CAD build for the part. Positions are in the model's coordinates, mm. Face numbers are marked on the shaded views. A direction names the side the tool comes from. Give positions to 0.01 mm unless a question says otherwise; leave off trailing zeros. Loops run counter-clockwise (first coordinate to the right, second up) from the corner with the lowest first, then second, coordinate; pieces in that order, holes last.
```python
from build123d import *

# Parameters (mm, degrees)
SKETCH1_R               = 15.875
BOSS_EXTRUDE1_DEPTH     = 9.2
SKETCH2_W               = 2.259426776
SKETCH2_H               = 16.292984729
SKETCH2_W_2             = 2.453909841
SKETCH2_H_2             = 18.61191006
CUT_EXTRUDE2_DEPTH      = 2
SKETCH3_R               = 4
BOSS_EXTRUDE3_DEPTH     = 1
BOSS_EXTRUDE4_START     = -5
BOSS_EXTRUDE4_OUTLINE_R = 1.7
BOSS_EXTRUDE4_DEPTH     = 5


# Read off the part's stored shape, not the designer's step: Boss-Extrude4
with BuildPart() as part:
    # Sketch1 → Boss-Extrude1 (new body)
    with BuildSketch(Plane(origin=(0, 0, 0), x_dir=(1, 0, 0), z_dir=(0, 1, 0))):
        with Locations(Location((0, 0, 0), (0, 0, 270))):
            Circle(SKETCH1_R)
    extrude(amount=BOSS_EXTRUDE1_DEPTH)

    # Sketch2 → Cut-Extrude2 (cut)
    with BuildSketch(Plane(origin=(0, 9.2, 0), x_dir=(1, 0, 0), z_dir=(0, 1, 0))):
        with Locations((-15.629713388, -0.847675915)):
            Rectangle(SKETCH2_W, SKETCH2_H)
        with Locations((15.726954921, -2.007138581)):
            Rectangle(SKETCH2_W_2, SKETCH2_H_2)
    extrude(amount=-CUT_EXTRUDE2_DEPTH, mode=Mode.SUBTRACT)

    # Sketch3 → Boss-Extrude3 (add)
    with BuildSketch(Plane(origin=(0, 9.2, 0), x_dir=(1, 0, 0), z_dir=(0, 1, 0))):
        with Locations(Location((0, 0, 0), (0, 0, 270))):
            Circle(SKETCH3_R)
    extrude(amount=BOSS_EXTRUDE3_DEPTH)

    # Boss-Extrude4 outline → Boss-Extrude4 (cut)
    with BuildSketch(Plane.XZ.offset(BOSS_EXTRUDE4_START)):
        with Locations((0, 12.7)):
            Circle(BOSS_EXTRUDE4_OUTLINE_R)
        with Locations((0, -12.7)):
            Circle(BOSS_EXTRUDE4_OUTLINE_R)
    extrude(amount=BOSS_EXTRUDE4_DEPTH, mode=Mode.SUBTRACT)


solid = part.part
```
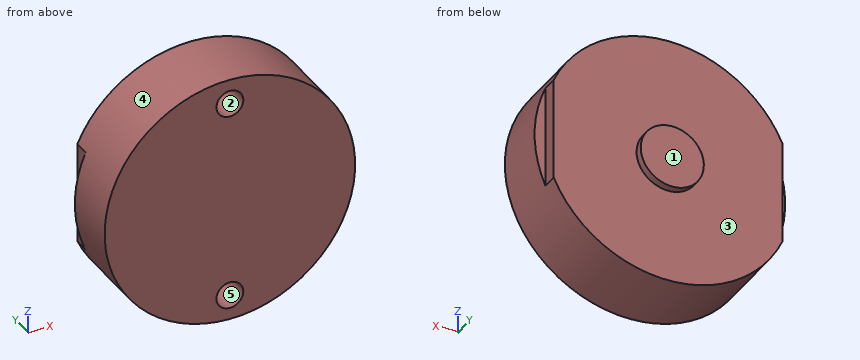
1. Saw through at B-B, the plane z = 13.5. List the corners of the cut face in (x, y).
Responses:
outline: (-8.35, 0) - (-1.5, 0) - (-1.5, 5) - (1.5, 5) - (1.5, 0) - (8.35, 0) - (8.35, 9.2) - (-8.35, 9.2) - close
2. Saw through at C-C, the plane y = 3. List the corners of the cut face in (x, z) (3 decimals).
Responses:
outline: circle Ø31.75 at (0, 0); hole circle Ø3.4 at (0, -12.7); hole circle Ø3.4 at (0, 12.7)
3. Saw through at A-A, the plane x = 0. List the corners of the cut face in (y, z) (3 decimals).
Responses:
outline: (0, -15.875) - (9.2, -15.875) - (9.2, -4) - (10.2, -4) - (10.2, 4) - (9.2, 4) - (9.2, 15.875) - (0, 15.875) - (0, 14.4) - (5, 14.4) - (5, 11) - (0, 11) - (0, -11) - (5, -11) - (5, -14.4) - (0, -14.4) - close
4. Pull direction Z, two halves, no side cores. Call the marked faces 3, 4 and 5: released by +Z, released by -Z, zero draft, split by the parting line, or undercut.
Responses:
face 3: zero draft
face 4: split by the parting line
face 5: undercut
5. Probe line 1 along Z through (x, y) = (0, 2.15) (3 decimals); line 2 along Y through (x, z) = (-4.5, 12); line 3 along Y through (x, z) = (0, 13). List the from-to ranges inside material, lowest first.
Responses:
line 1: z = -15.875 to -14.4, -11 to 11, 14.4 to 15.875
line 2: y = 0 to 9.2
line 3: y = 5 to 9.2
6. Saw through at D-D, the plane y = 6.25. List the corners of the cut face in (x, z) (3 decimals).
Responses:
outline: circle Ø31.75 at (0, 0)
7. Tool access for the marked faces 1 and 2: list every direction of +Z, -Z, +X, -X, +Y, -Y with a clear straight run to the whole face (end or side of a thin tool).
Responses:
face 1: +Z, -Z, +X, -X, +Y
face 2: -Y
8. Drop flat-ended pins along their axis: pin 1 (3 mm diameter, centred on y = 2, z = 11, fed in from +X); pin 2 (2 mm diameter, centred on x = 0, z = 12.7, fed in from -Y); pin 3 (1.5 mm diameter, centred on x = 6.5, y = 7.5, fed in from -Z). Give the stop position or say it passes through.
Responses:
pin 1: stops at x = 12.72
pin 2: stops at y = 5
pin 3: stops at z = -14.8
